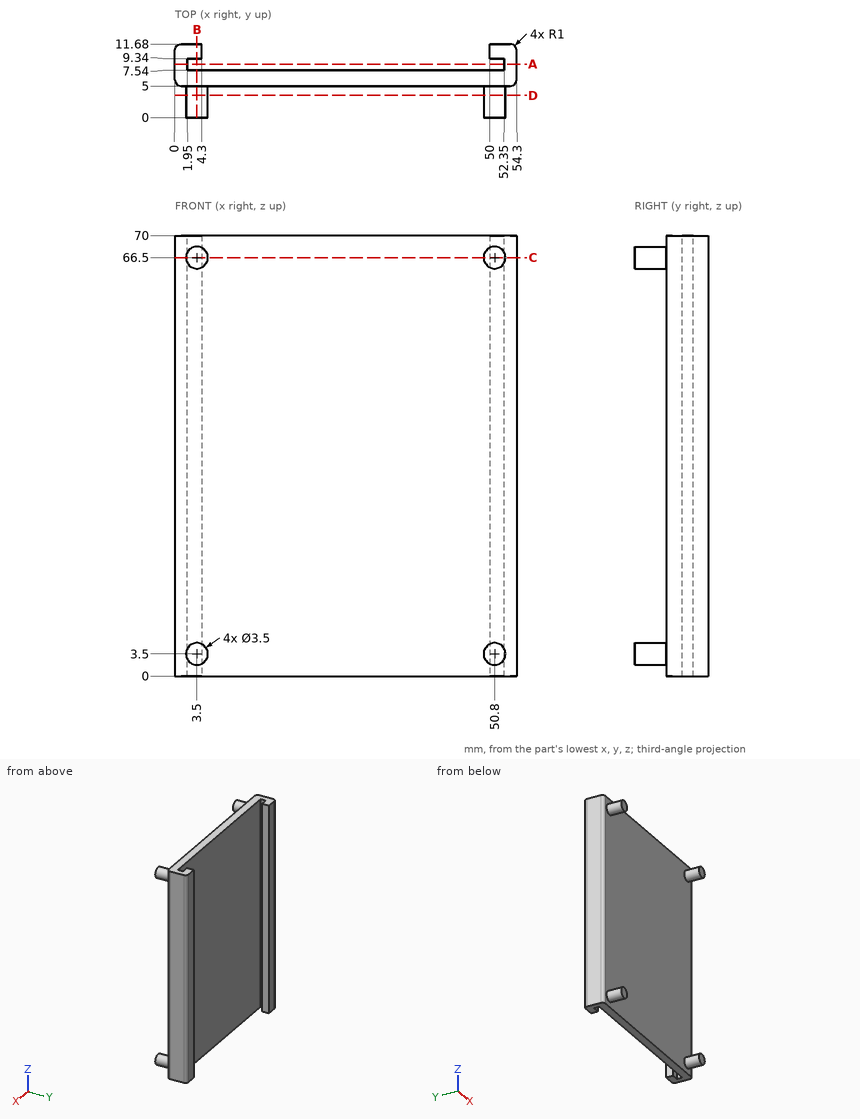
Print and shaded views of the part. All mm, measured from the part's lowest x, y and z. Coordinates: 2 decimals unless noted, no trailing zeros. Order: outer loops, then holes, each group sorted by start corner. A loop starts at its lowest first (then second) coordinate and runs counter-clockwise, first axis right, second up.
(1) Probe L1, parallel to X at y = 9, z = 30; L2, parallel to Y at x = 47, z = 62; L3, parallel to X at y = 3, z = 3. List the from-to ranges inside material, lowest first.
Check sheet entries:
L1: x = 0 to 1.95, 52.35 to 54.3
L2: y = 5 to 7.54
L3: x = 1.82 to 5.18, 49.12 to 52.48
(2) Pin check, flat tips, straight feed: pin 1 Ø0.9 at (y, z) = (8.5, 33.5) entering from -X; pin 2 Ø1.5 at (x, y) = (24, 4) entering from -Z; pin 3 Ø15.5 at (x, z) = (37, 19.5) entering from -Y; pin 4 Ø12 at (x, z) = (38, 19) entering from +Y. Stop position of each tip, or through.
Check sheet entries:
pin 1: stops at x = 0
pin 2: passes through
pin 3: stops at y = 5
pin 4: stops at y = 7.54
(3) Slice it at A-A, the plane y = 8.5. Write the cut outline in (x, z).
Check sheet entries:
outline: (0, 0) - (1.95, 0) - (1.95, 70) - (0, 70) - close; (52.35, 0) - (54.3, 0) - (54.3, 70) - (52.35, 70) - close
(4) Slice it at B-B, the plane x = 3.5. Write the cut outline in (y, z), and give its area (3 significant figures).
Check sheet entries:
outline: (0, 1.75) - (5, 1.75) - (5, 0) - (7.54, 0) - (7.54, 70) - (5, 70) - (5, 68.25) - (0, 68.25) - (0, 64.75) - (5, 64.75) - (5, 5.25) - (0, 5.25) - close; (9.34, 0) - (11.68, 0) - (11.68, 70) - (9.34, 70) - close
area: 377 mm2
(5) Slice it at D-D, the plane y = 3.5. Write the cut outline in (x, z), and give its area (3 significant figures).
Check sheet entries:
outline: circle Ø3.5 at (3.5, 3.5); circle Ø3.5 at (3.5, 66.5); circle Ø3.5 at (50.8, 3.5); circle Ø3.5 at (50.8, 66.5)
area: 38.5 mm2
(6) Slice it at C-C, the plane z = 66.5. Write the cut outline in (x, y), and give its area (3 significant figures).
Check sheet entries:
outline: (0, 6) arc R1 ccw to (1, 5) - (1.75, 5) - (1.75, 0) - (5.25, 0) - (5.25, 5) - (49.05, 5) - (49.05, 0) - (52.55, 0) - (52.55, 5) - (53.3, 5) arc R1 ccw to (54.3, 6) - (54.3, 10.68) arc R1 ccw to (53.3, 11.68) - (50, 11.68) - (50, 9.34) - (52.35, 9.34) - (52.35, 7.54) - (1.95, 7.54) - (1.95, 9.34) - (4.3, 9.34) - (4.3, 11.68) - (1, 11.68) arc R1 ccw to (0, 10.68) - close
area: 199 mm2
